The model under review builds one solid part; all positions refer to its coordinate system, in mm. Coordinates: 2 decimals unless noted, no trailing zeros. Order: outer loops, then holes, each group sorted by start corner. A loop starts at its lowest first (then second) coordinate and runs counter-clockwise, first axis right, second up.
```python
from build123d import *

# Parameters (mm, degrees)
SKETCH_1_W      = 29
SKETCH_1_H      = 12.7
EXTRUDE_1_DEPTH = 15.7
EXTRUDE_2_DEPTH = 3.5
FILLET_1_R      = 0.05
CHAMFER_1_SIZE  = 1.5
FILLET_2_R      = 0.75


with BuildPart() as part:
    # Эскиз1 → Бобышка-Вытянуть1 (new body)
    with BuildSketch(Plane(origin=(0, 0, 0), x_dir=(1, 0, 0), z_dir=(0, 1, 0))):
        Rectangle(SKETCH_1_W, SKETCH_1_H)
    extrude(amount=EXTRUDE_1_DEPTH)

    # Эскиз2 → Бобышка-Вытянуть2 (add)
    with BuildSketch(Plane.XZ):
        with BuildLine():
            Line((-12.3, 4.15), (-11.9, 4.15))
            ThreePointArc((-11.9, 4.15), (-11.864644661, 4.135355339), (-11.85, 4.1))
            Line((-11.85, 4.1), (-11.85, 3.4))
            ThreePointArc((-11.85, 3.4), (-11.864644661, 3.364644661), (-11.9, 3.35))
            Line((-11.9, 3.35), (-12.3, 3.35))
            ThreePointArc((-12.3, 3.35), (-12.335355339, 3.364644661), (-12.35, 3.4))
            Line((-12.35, 3.4), (-12.35, 4.1))
            ThreePointArc((-12.35, 4.1), (-12.335355339, 4.135355339), (-12.3, 4.15))
        make_face()
        with BuildLine():
            Line((7.65, -3.4), (7.65, -4.1))
            ThreePointArc((7.65, -4.1), (7.664644661, -4.135355339), (7.7, -4.15))
            Line((7.7, -4.15), (8.1, -4.15))
            ThreePointArc((8.1, -4.15), (8.135355339, -4.135355339), (8.15, -4.1))
            Line((8.15, -4.1), (8.15, -3.4))
            ThreePointArc((8.15, -3.4), (8.135355339, -3.364644661), (8.1, -3.35))
            Line((8.1, -3.35), (7.7, -3.35))
            ThreePointArc((7.7, -3.35), (7.664644661, -3.364644661), (7.65, -3.4))
        make_face()
        with BuildLine():
            Line((-12.35, -3.4), (-12.35, -4.1))
            ThreePointArc((-12.35, -4.1), (-12.335355339, -4.135355339), (-12.3, -4.15))
            Line((-12.3, -4.15), (-11.9, -4.15))
            ThreePointArc((-11.9, -4.15), (-11.864644661, -4.135355339), (-11.85, -4.1))
            Line((-11.85, -4.1), (-11.85, -3.4))
            ThreePointArc((-11.85, -3.4), (-11.864644661, -3.364644661), (-11.9, -3.35))
            Line((-11.9, -3.35), (-12.3, -3.35))
            ThreePointArc((-12.3, -3.35), (-12.335355339, -3.364644661), (-12.35, -3.4))
        make_face()
        with BuildLine():
            Line((11.2, 4.15), (11.6, 4.15))
            ThreePointArc((11.6, 4.15), (11.635355339, 4.135355339), (11.65, 4.1))
            Line((11.65, 4.1), (11.65, 3.4))
            ThreePointArc((11.65, 3.4), (11.635355339, 3.364644661), (11.6, 3.35))
            Line((11.6, 3.35), (11.2, 3.35))
            ThreePointArc((11.2, 3.35), (11.164644661, 3.364644661), (11.15, 3.4))
            Line((11.15, 3.4), (11.15, 4.1))
            ThreePointArc((11.15, 4.1), (11.164644661, 4.135355339), (11.2, 4.15))
        make_face()
    extrude(amount=EXTRUDE_2_DEPTH)

    # Скругление1
    fillet_1_edges = [part.edges().sort_by_distance(p)[0] for p in [
        (-12.335355339, -3.5, 3.364644661),
        (-12.1, -3.5, 3.35),
        (-11.864644661, -3.5, 3.364644661),
        (-11.85, -3.5, 3.75),
        (-11.864644661, -3.5, 4.135355339),
        (-12.1, -3.5, 4.15),
        (-12.335355339, -3.5, 4.135355339),
        (-12.35, -3.5, 3.75),
        (7.664644661, -3.5, -4.135355339),
        (7.9, -3.5, -4.15),
        (8.135355339, -3.5, -4.135355339),
        (8.15, -3.5, -3.75),
        (8.135355339, -3.5, -3.364644661),
        (7.9, -3.5, -3.35),
        (7.664644661, -3.5, -3.364644661),
        (7.65, -3.5, -3.75),
        (-12.335355339, -3.5, -4.135355339),
        (-12.1, -3.5, -4.15),
        (-11.864644661, -3.5, -4.135355339),
        (-11.85, -3.5, -3.75),
        (-11.864644661, -3.5, -3.364644661),
        (-12.1, -3.5, -3.35),
        (-12.335355339, -3.5, -3.364644661),
        (-12.35, -3.5, -3.75),
    ]]
    fillet(fillet_1_edges, radius=FILLET_1_R)

    # Фаска1
    chamfer_1_edges = [part.edges().sort_by_distance(p)[0] for p in [
        (14.5, 15.7, 0),
    ]]
    chamfer(chamfer_1_edges, length=CHAMFER_1_SIZE)

    # Скругление2
    fillet_2_edges = [part.edges().sort_by_distance(p)[0] for p in [
        (-14.5, 15.7, 0),
        (-0.75, 15.7, 6.35),
        (-0.75, 15.7, -6.35),
        (13, 15.7, 0),
        (14.5, 7.1, -6.35),
        (13.75, 14.95, -6.35),
        (14.5, 7.1, 6.35),
        (14.5, 14.2, 0),
        (13.75, 14.95, 6.35),
        (-14.5, 7.85, 6.35),
        (-14.5, 7.85, -6.35),
    ]]
    fillet(fillet_2_edges, radius=FILLET_2_R)


solid = part.part
```
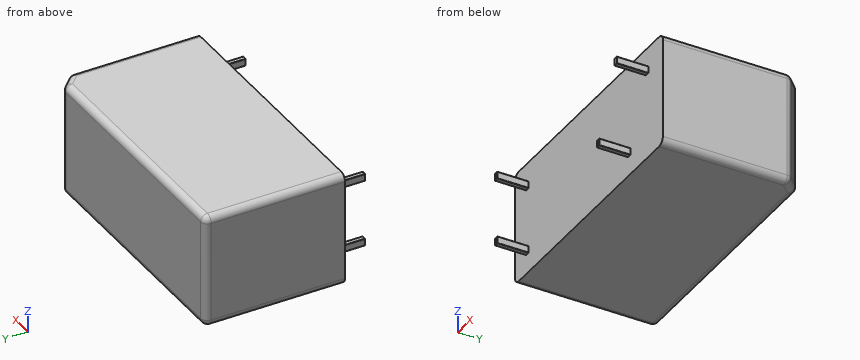
(1) Wall thickness on probe 1 along Y at (x, z) = (11, 0.25); probe 2 along X at (y, z) = (14, 5); probe 3 along X at (y, z) = (14.5, -1.25): over which ranges is each line inside the solid? List them lowest first.
A:
probe 1: y = 0 to 15.7
probe 2: x = -14.5 to 14.49
probe 3: x = -14.5 to 14.2
(2) We need section A-A, the plane y = -2. Count the separate pieces of the cut face and the enclosed holes in it, and give its area (3 significant figures).
A:
separate pieces: 4
enclosed holes: 0
area: 1.59 mm2
(3) We need section C-C, the plane x = 3.75. Write out the cut boundary in (y, z), and give its area (3 significant figures).
A:
outline: (0, -6.35) - (14.95, -6.35) arc R0.75 ccw to (15.7, -5.6) - (15.7, 5.6) arc R0.75 ccw to (14.95, 6.35) - (0, 6.35) - close
area: 199 mm2
(4) We need section B-B, the plane z = -2.5. Write out the cut boundary in (x, y).
A:
outline: (-14.5, 0) - (14.5, 0) - (14.5, 13.89) arc R0.75 ccw to (14.28, 14.42) - (13.22, 15.48) arc R0.75 ccw to (12.69, 15.7) - (-13.75, 15.7) arc R0.75 ccw to (-14.5, 14.95) - close
(5) For pin 1 Ø0.8 at (y, z) = (-1.5, -4) entering from -X; pin 2 Ø0.8 at (y, z) = (-1, -4) entering from +X; pin 3 Ø4 at (x, z) = (5, 0) entering from -Y, all flat-tipped, find the tip position at first contact; note any pin that passes through.
A:
pin 1: stops at x = -12.35
pin 2: stops at x = 8.15
pin 3: stops at y = 0
